from build123d import *


with BuildPart() as part:
    # Sweep1: sweep along a path in Sketch2
    with BuildLine(Plane(origin=(0, 0, 0), x_dir=(1, 0, 0), z_dir=(0, 1, 0))) as sweep1_path:
        Line((-374.65, 0), (-374.65, -361.95))
        Line((-374.65, -361.95), (374.65, -361.95))
        Line((374.65, -361.95), (374.65, 0))
    # Sketch1 → Sweep1 (sweep)
    with BuildSketch(Plane.XY):
        with BuildLine():
            Line((-393.7, 127), (-425.45, 127))
            ThreePointArc((-425.45, 127), (-447.900640303, 117.700640303), (-457.2, 95.25))
            Line((-457.2, 95.25), (-457.2, 31.75))
            ThreePointArc((-457.2, 31.75), (-447.900640303, 9.299359697), (-425.45, 0))
            Line((-425.45, 0), (-393.7, 0))
            Line((-393.7, 0), (-374.65, 0))
            Line((-374.65, 0), (-374.65, 127))
            Line((-374.65, 127), (-393.7, 127))
        make_face()
    sweep(path=sweep1_path.line, transition=Transition.RIGHT)


solid = part.part
Input: part model. Units: mm. Frame: model coordinates. A direction names the side the tool comes from. Give positions to 0.01 mm unless a question says otherwise; leave off trailing zeros. Write each loop counter-clockwise with the first axis right and the second up, starting at its lowest first coordinate (ties: lowest second). Pieces come first, ordered by that corner, then holes. Notation, with made-up numbers: (-14.75, -7.5) -> (36.25, -7.5) arc R17 cw to (36.25, 12.5) -> close; hole circle Ø8 at (-25, 67). An arc over 180 degrees is marked (long way). Use one line per item in the form item = value. Start each with the question number.
1) Draft query along X for faces 3 (the cylindrical face through (448.1, 9.5, 219.1)), 4 (the flat face through (374.65, 63, 178)), 5 (the cylindrical face through (6.4, 117.9, 435)). Return one class per face: pulls with the +X half, pulls with the -X half, needs draft (parallel to the pull), parting line crosses it, or undercut.
2) Pin query (flat end, axial travel): pin 1 (1.5 mm diameter, centred on x = -235, y = 68.5, fed in from -Z); pin 2 (1 mm diameter, centred on x = -2.5, y = 97.5, fed in from +Z). Return the tip coordinate at first contact, or that it passes through.
3) Section query C-C on x = 123.5. Return the cut outline in (y, z), then the cut area to 3 significant figures.
4) Section query A-A on z = 260. Return the cut outline in (x, y).
5) Section query D-D on y = 118.5. Return the cut outline in (x, z).
6) Ray query, probe 1 along X at (y, z) = (44, 99); probe 2 along X at (y, z) = (26.5, 168); probe 3 along Y at (x, z) = (351, 414). Return the intervals inside material, ascending. Write a range as from..to.
7) Set-up query: faces 1 (the flat face through (-457.2, 64, 225)), 2 (the flat face through (-374.65, 63, 184)). Return all of +Z, -Z, +X, -X, +Y, -Y with unobstructed straight access to the full face (end or side cutting, diameter ignored); none if empty.
8) Section query B-B on y = 67. Return the cut outline in (x, z).
Outcome:
q1.face_3 = pulls with the +X half
q1.face_4 = undercut
q1.face_5 = needs draft
q2.pin_1 = 361.95
q2.pin_2 = 444.45
q3.outline = (0, 361.95) -> (127, 361.95) -> (127, 412.75) arc R31.75 ccw to (95.25, 444.5) -> (31.75, 444.5) arc R31.75 ccw to (0, 412.75) -> close
q3.area = 10,100 mm^2
q4.outline = (-457.2, 31.75) arc R31.75 ccw to (-425.45, 0) -> (-374.65, 0) -> (-374.65, 127) -> (-425.45, 127) arc R31.75 ccw to (-457.2, 95.25) -> close; (374.65, 0) -> (425.45, 0) arc R31.75 ccw to (457.2, 31.75) -> (457.2, 95.25) arc R31.75 ccw to (425.45, 127) -> (374.65, 127) -> close
q5.outline = (-447.07, 0) -> (-374.65, 0) -> (-374.65, 361.95) -> (374.65, 361.95) -> (374.65, 0) -> (447.07, 0) -> (447.07, 434.37) -> (-447.07, 434.37) -> close
q6.probe_1 = -457.2..-374.65, 374.65..457.2
q6.probe_2 = -456.76..-374.65, 374.65..456.76
q6.probe_3 = 0.02..126.98
q7.face_1 = +Z, -Z, -X, +Y, -Y
q7.face_2 = -Z, +Y, -Y
q8.outline = (-457.2, 0) -> (-374.65, 0) -> (-374.65, 361.95) -> (374.65, 361.95) -> (374.65, 0) -> (457.2, 0) -> (457.2, 444.5) -> (-457.2, 444.5) -> close
